Read the model definition and answer for the solid it produces. Units are mm, in the model's axes. A direction names the side the tool comes from. Coordinates: 2 decimals unless noted, no trailing zeros. Loops run counter-clockwise (first coordinate to the right, second up) from the corner with the lowest first, then second, coordinate; pieces in that order, holes last.
from build123d import *

# Parameters (mm, degrees)
F2_W     = 68
F2_H     = 45
F3_DEPTH = 29.5
F4_R     = 15
F5_T     = -1.25
F6_DEPTH = 0.35


with BuildPart() as f3:
    # F2 (on Top) → F3 (new body)
    with BuildSketch(Plane.XY):
        Rectangle(F2_W, F2_H)
    extrude(amount=F3_DEPTH)

    # F4
    f4_edges = [f3.edges().sort_by_distance(p)[0] for p in [
        (34, -22.5, 14.75),
        (34, 22.5, 14.75),
        (-34, -22.5, 14.75),
        (-34, 22.5, 14.75),
    ]]
    fillet(f4_edges, radius=F4_R)

    # F5
    f5_openings = [f3.faces().sort_by_distance(p)[0] for p in [
        (0, 0, 29.5),
    ]]
    offset(amount=F5_T, openings=f5_openings)

    # F6 (cut): a face of the model
    f6_faces = [f3.faces().sort_by_distance(p)[0] for p in [
        (0, 0, 1.25),
    ]]
    extrude(f6_faces, amount=-F6_DEPTH, mode=Mode.SUBTRACT)


solid = f3.part
Item 1: A cutting plane is placed at A-A on z = 8. Determine the outline of the cut face in (x, y).
Numbers:
outline: (-34, -7.5) arc R15 ccw to (-19, -22.5) - (19, -22.5) arc R15 ccw to (34, -7.5) - (34, 7.5) arc R15 ccw to (19, 22.5) - (-19, 22.5) arc R15 ccw to (-34, 7.5) - close; hole (-32.75, -7.5) arc R13.75 ccw to (-19, -21.25) - (19, -21.25) arc R13.75 ccw to (32.75, -7.5) - (32.75, 7.5) arc R13.75 ccw to (19, 21.25) - (-19, 21.25) arc R13.75 ccw to (-32.75, 7.5) - close
Item 2: Find the intervals of material crossed by line 1 along X through (y, z) = (2.5, 2.75); line 2 along Y through (x, z) = (9, 24.5); line 3 along X through (y, z) = (8, 17.25), in increasing order.
Numbers:
line 1: x = -34 to -32.75, 32.75 to 34
line 2: y = -22.5 to -21.25, 21.25 to 22.5
line 3: x = -33.99 to -32.74, 32.74 to 33.99
Item 3: Which of the six approach directions +Z, -Z, +X, -X, +Y, -Y give full straight-line access (tool end or side, diameter ignored) to faces 4 (the face through (-32.75, 0, 15)), 5 (the face through (29.49, -18.22, 14.96))?
Numbers:
face 4: +Z
face 5: +Z, -Z, +X, -Y
Item 4: Given pin 1 (8 mm diameter, centred on x = -9.5, y = -16.5, fed in from +Z), flat-ended and moving along its own axis, determine where the tip first touches the part or whether it passes through.
Numbers:
pin 1: stops at z = 0.9
Item 5: A cutting plane is placed at B-B on y = -2. Determine the outline of the cut face in (x, z), then the cut area to 3 significant figures.
Numbers:
outline: (-34, 0) - (34, 0) - (34, 29.5) - (32.75, 29.5) - (32.75, 0.9) - (-32.75, 0.9) - (-32.75, 29.5) - (-34, 29.5) - close
area: 133 mm2
Item 6: A cutting plane is placed at C-C on x = -15. Determine the outline of the cut face in (y, z).
Numbers:
outline: (-22.5, 0) - (22.5, 0) - (22.5, 29.5) - (21.25, 29.5) - (21.25, 0.9) - (-21.25, 0.9) - (-21.25, 29.5) - (-22.5, 29.5) - close
Item 7: Determine the mould class of faces 1 (the face through (-34, 0, 15)), 2 (the face through (34, 0, 15)), 3 (the face through (28.615, -17.329, 15.4)) for opening direction X: released by +X, released by -X, zero draft, split by the parting line, or undercut.
Numbers:
face 1: released by -X
face 2: released by +X
face 3: undercut
